from build123d import *

# Parameters (mm, degrees)
ESTRUSIONE_ESTRUSIONE2_DEPTH = 200
SCHIZZO2_W                   = 6.628026169
SCHIZZO2_H                   = 20
ESTRUSIONE_ESTRUSIONE3_DEPTH = 200
RACCORDO3_R                  = 15


with BuildPart() as part:
    # Schizzo1 → Estrusione-Estrusione2 (new body)
    with BuildSketch(Plane.XY):
        with BuildLine():
            Line((-39.628026169, 0), (-33, 0))
            ThreePointArc((-33, 0), (0, 33), (33, 0))
            Line((33, 0), (39.628026169, 0))
            ThreePointArc((39.628026169, 0), (0, 39.628026169), (-39.628026169, 0))
        make_face()
    extrude(amount=ESTRUSIONE_ESTRUSIONE2_DEPTH)

    # Schizzo2 → Estrusione-Estrusione3 (add)
    with BuildSketch(Plane.XY):
        with Locations((-36.314013085, -10)):
            Rectangle(SCHIZZO2_W, SCHIZZO2_H)
        with Locations((36.314013085, -10)):
            Rectangle(SCHIZZO2_W, SCHIZZO2_H)
    extrude(amount=ESTRUSIONE_ESTRUSIONE3_DEPTH)

    # Raccordo3
    raccordo3_edges = [part.edges().sort_by_distance(p)[0] for p in [
        (-36.314013085, -20, 0),
        (-36.314013085, -20, 200),
        (36.314013085, -20, 0),
        (36.314013085, -20, 200),
    ]]
    fillet(raccordo3_edges, radius=RACCORDO3_R)


solid = part.part
Design review of the part built by this model. Coordinates are the model's own, in mm. A direction names the side the tool comes from. Coordinates: 2 decimals unless noted, no trailing zeros. Order: outer loops, then holes, each group sorted by start corner. A loop starts at its lowest first (then second) coordinate and runs counter-clockwise, first axis right, second up. Notation, with made-up numbers: (-24.75, -8) - (9.25, -8) arc R20 cw to (9.25, 10) - close; hole circle Ø5 at (88, -2). An arc over 180 degrees is marked (long way). Put each result on its own line as item: value.
1) Take a section at C-C, the plane x = -8. Give the boundary of the cut face in (y, z), and give its area (3 significant figures).
Response values:
outline: (32.02, 0) - (38.81, 0) - (38.81, 200) - (32.02, 200) - close
area: 1,360 mm²
2) Take a section at A-A, the plane z = 156.5. Give the boundary of the cut face in (x, y), and give its area (3 significant figures).
Response values:
outline: (-39.63, -20) - (-33, -20) - (-33, 0) arc R33 cw to (33, 0) - (33, -20) - (39.63, -20) - (39.63, 0) arc R39.63 ccw to (-39.63, 0) - close
area: 1,020 mm²
3) Take a section at D-D, the plane y = 11.5. Give the boundary of the cut face in (x, z), and give its area (3 significant figures).
Response values:
outline: (-37.92, 0) - (-30.93, 0) - (-30.93, 200) - (-37.92, 200) - close; (30.93, 0) - (37.92, 0) - (37.92, 200) - (30.93, 200) - close
area: 2,800 mm²
4) Wall thickness on L1, parallel to X at y = -5.5, z = 120.5; L2, parallel to X at y = 5.5, z = 129; L3, parallel to Y at x = -17, z = 74: over which ranges is each line inside the solid? List them lowest first. Write a range as from..to.
Response values:
L1: x = -39.63..-33, 33..39.63
L2: x = -39.24..-32.54, 32.54..39.24
L3: y = 28.28..35.8
5) The part is to be moulded in two halves that separate along X. For faces 3 (the face through (-39.628, -10, 99)), 4 (the face through (-33, -10, 99)), 5 (the face through (39.628, -10, 99)), say which applies: released by +X, released by -X, zero draft, split by the parting line, or undercut.
Response values:
face 3: released by -X
face 4: undercut
face 5: released by +X
6) Tool access review of faces 1 (the face through (-36.27, -15.72, 195.49)), 2 (the face through (33, -10, 99)): name each direction out of +Z, -Z, +X, -X, +Y, -Y from which nothing blocks a thin tool from reaching the whole face with its end or side.
Response values:
face 1: +Z, +X, -X, -Y
face 2: +Z, -Z, -Y
7) Insertion check: P1, Ø5, axis at y = 27.5, z = 118, coming from the -X side; P2, Ø12, axis at x = 17, z = 149.5, coming from the +Y side; P3, Ø12, axis at y = 21, z = 103.5, coming from the +X side; P4, Ø8, axis at x = -11, y = 22.5, coming from the +Z side. Each pin has a flat end and moves straight along its axis. Give the tip position at first contact, or say it passes through.
Response values:
P1: stops at x = -30.75
P2: stops at y = 38.07
P3: stops at x = 36.68
P4: passes through
8) Take a section at B-B, the plane y = 2. Give the boundary of the cut face in (x, z).
Response values:
outline: (-39.58, 0) - (-32.94, 0) - (-32.94, 200) - (-39.58, 200) - close; (32.94, 0) - (39.58, 0) - (39.58, 200) - (32.94, 200) - close
